Input: part model. Units: mm. Frame: model coordinates. A direction names the side the tool comes from. Give positions to 0.01 mm unless a question says otherwise; leave off trailing zeros. Loops run counter-clockwise (first coordinate to the right, second up) from the corner with the lowest first, then second, coordinate; pieces in that order, holes last. Notation, with made-up numbers: (-31.75, -10.5) -> (-10.75, -10.5) arc R26 ccw to (-10.75, 10.5) -> close; hole circle Ø5 at (35.25, 68.5). An arc over 180 degrees is marked (long way). Answer as a JSON object with one key per item and string values.
```python
from build123d import *

# Parameters (mm, degrees)
F0_R     = 10.9982
F1_DEPTH = 6.35
F2_R     = 2.54


with BuildPart() as f1:
    # F0 (on Top) → F1 (new body)
    with BuildSketch(Plane.XY):
        with BuildLine():
            ThreePointArc((-44.45, 0), (-38.4948291982, -22.225), (-22.225, -38.4948291982))
            Line((-22.225, -38.4948291982), (-8.89, -15.3979316793))
            ThreePointArc((-8.89, -15.3979316793), (-15.3979316793, -8.89), (-17.78, 0))
            Line((-17.78, 0), (-44.45, 0))
        make_face()
        with Locations((-26.1790094785, -15.6166254914)):
            Circle(F0_R, mode=Mode.SUBTRACT)
        with BuildLine():
            Line((8.89, 15.3979316793), (22.225, 38.4948291982))
            ThreePointArc((22.225, 38.4948291982), (0, 44.45), (-22.225, 38.4948291982))
            Line((-22.225, 38.4948291982), (-8.89, 15.3979316793))
            ThreePointArc((-8.89, 15.3979316793), (0, 17.78), (8.89, 15.3979316793))
        make_face()
        with Locations((-0.4348896577, 30.48)):
            Circle(F0_R, mode=Mode.SUBTRACT)
        with BuildLine():
            ThreePointArc((22.225, -38.4948291982), (38.4948291982, -22.225), (44.45, 0))
            Line((44.45, 0), (17.78, 0))
            ThreePointArc((17.78, 0), (15.3979316793, -8.89), (8.89, -15.3979316793))
            Line((8.89, -15.3979316793), (22.225, -38.4948291982))
        make_face()
        with Locations((26.6138991362, -14.8633745086)):
            Circle(F0_R, mode=Mode.SUBTRACT)
        with BuildLine():
            ThreePointArc((8.89, -15.3979316793), (15.3979316793, -8.89), (17.78, 0))
            ThreePointArc((17.78, 0), (15.3979316793, 8.89), (8.89, 15.3979316793))
            ThreePointArc((8.89, 15.3979316793), (0, 17.78), (-8.89, 15.3979316793))
            ThreePointArc((-8.89, 15.3979316793), (-15.3979316793, 8.89), (-17.78, 0))
            ThreePointArc((-17.78, 0), (-15.3979316793, -8.89), (-8.89, -15.3979316793))
            ThreePointArc((-8.89, -15.3979316793), (0, -17.78), (8.89, -15.3979316793))
        make_face()
        Circle(F0_R, mode=Mode.SUBTRACT)
    extrude(amount=F1_DEPTH)

    # F2
    f2_edges = [f1.edges().sort_by_distance(p)[0] for p in [
        (-38.494829, -22.225, 6.35),
        (-15.5575, -26.94638, 6.35),
        (0, -17.78, 6.35),
        (15.5575, -26.94638, 6.35),
        (38.494829, -22.225, 6.35),
        (31.115, 0, 6.35),
        (15.397932, 8.89, 6.35),
        (15.5575, 26.94638, 6.35),
        (0, 44.45, 6.35),
        (-15.5575, 26.94638, 6.35),
        (-15.397932, 8.89, 6.35),
        (-31.115, 0, 6.35),
        (-15.5575, 26.94638, 0),
        (0, 44.45, 0),
        (15.5575, 26.94638, 0),
        (38.494829, -22.225, 0),
        (31.115, 0, 0),
        (15.5575, -26.94638, 0),
        (-15.397932, 8.89, 0),
        (15.397932, 8.89, 0),
        (-31.115, 0, 0),
        (-38.494829, -22.225, 0),
        (-15.5575, -26.94638, 0),
        (0, -17.78, 0),
    ]]
    fillet(f2_edges, radius=F2_R)


solid = f1.part
```
Q1. Pin query (flat end, axial travel): pin 1 (1 mm diameter, centred on x = 31.5, z = 3.5, fed in from +Y); pin 2 (2 mm diameter, centred on y = 12, z = 3.5, fed in from -X). Return the tip coordinate at first contact, or that it passes through.
Evaluation:
{"pin 1": "stops at y = 0", "pin 2": "stops at x = -13.97"}
Q2. Access query for faces 1 (the cylindrical face through (-14.1, 25.9, 5.6)), 2 (the cylindrical face through (15.599, -25.57, 5.586)), 3 (the cylindrical face through (29.532, -0.724, 5.586)), 4 (the flat face through (-15.65, 27.11, 3.17)). Directions: +Z, -Z, +X, -X, +Y, -Y. A direction counts if a zero-diameter tool reaches every point of the face in a straight line with its end or side. Return the directions, or none.
Evaluation:
{"face 1": "+Z, -X", "face 2": "+Z, -Y", "face 3": "+Z, +X", "face 4": "+Z, -Z, -X"}
Q3. Section A-A, the plane x = 0. Return the cut outline in (y, z), then the cut area to 3 significant figures.
Evaluation:
{"outline": "(-17.78, 2.54) arc R2.54 ccw to (-15.24, 0) -> (-11, 0) -> (-11, 6.35) -> (-15.24, 6.35) arc R2.54 ccw to (-17.78, 3.81) -> close; (11, 0) -> (19.49, 0) -> (19.49, 6.35) -> (11, 6.35) -> close; (41.47, 0) -> (41.91, 0) arc R2.54 ccw to (44.45, 2.54) -> (44.45, 3.81) arc R2.54 ccw to (41.91, 6.35) -> (41.47, 6.35) -> close", "area": "110 mm2"}
Q4. Draft query along X for faces 5 (the cylindrical face through (-14.139, 25.938, 0.764)), 6 (the cylindrical face through (14.34, 26.29, 5.59)), 7 (the flat face through (-15.65, -27.11, 3.17)), 8 (the cylindrical face through (0.33, 44.45, 3.17)). Return one class per face: +X half, -X half, draft (parallel to the pull), parting line (faces both ways), or undercut.
Evaluation:
{"face 5": "-X half", "face 6": "+X half", "face 7": "undercut", "face 8": "parting line"}
Q5. Section C-C, the plane y = -8.5. Give the number of separate pieces and of enclosed holes in the cut face, then the cut area to 3 significant figures.
Evaluation:
{"separate pieces": "4", "enclosed holes": "0", "area": "239 mm2"}
Q6. Ray query, line 1 along Y through (x, z) = (-1, 1); line 2 along Y through (x, z) = (-3, 1.75); line 3 along X through (y, z) = (-6.5, 1). Return the intervals inside material, ascending.
Evaluation:
{"line 1": "y = -17.23 to -10.95, 10.95 to 19.5, 41.46 to 43.92", "line 2": "y = -17.4 to -10.58, 10.58 to 19.79, 41.17 to 44.22", "line 3": "x = -43.45 to -32.33, -20.03 to -8.87, 8.87 to 19.47, 33.76 to 43.45"}
Q7. Section B-B, the plane z = 1.5. Return the cut outline in (x, y).
Evaluation:
{"outline": "(-44.23, -0.22) arc R44.23 ccw to (-22.31, -38.19) -> (-8.97, -15.09) arc R17.56 ccw to (8.97, -15.09) -> (22.31, -38.19) arc R44.23 ccw to (44.23, -0.22) -> (17.56, -0.22) arc R17.56 ccw to (8.59, 15.32) -> (21.92, 38.41) arc R44.23 ccw to (-21.92, 38.41) -> (-8.59, 15.32) arc R17.56 ccw to (-17.56, -0.22) -> close; hole circle Ø22 at (-26.18, -15.62); hole circle Ø22 at (-0.43, 30.48); hole circle Ø22 at (0, 0); hole circle Ø22 at (26.61, -14.86)"}
